```python
from build123d import *

# Parameters (mm, degrees)
SKETCH1_R                                            = 37.5
BOSS_EXTRUDE1_DEPTH                                  = 10
CSK_FOR_M6_HEX_SOCKET_COUNTERSUNK_CAP_SC_D           = 7
CSK_FOR_M6_HEX_SOCKET_COUNTERSUNK_CAP_SC_DEPTH       = 14.44
CSK_FOR_M6_HEX_SOCKET_COUNTERSUNK_CAP_SC_CSINK_D     = 13.44
CSK_FOR_M6_HEX_SOCKET_COUNTERSUNK_CAP_SC_CSINK_ANGLE = 90
CSK_FOR_M6_HEX_SOCKET_COUNTERSUNK_CAP_SC_TIP         = 2.103012167
SKETCH6_W                                            = 15
SKETCH6_H                                            = 30
BOSS_EXTRUDE2_DEPTH                                  = 7
SKETCH7_W                                            = 15
SKETCH7_H                                            = 30
BOSS_EXTRUDE3_DEPTH                                  = 7
BOSS_EXTRUDE4_START                                  = -7.5
BOSS_EXTRUDE4_DEPTH                                  = 7.5
FILLET1_R                                            = 10
SKETCH9_R                                            = 2.1
CUT_EXTRUDE1_DEPTH                                   = 6
SKETCH11_R                                           = 2.1
BOSS_EXTRUDE5_DEPTH                                  = 25
SKETCH12_W                                           = 3.472021997
SKETCH12_H                                           = 10.744400241
CUT_EXTRUDE2_DEPTH                                   = 25
BOSS_EXTRUDE7_DEPTH                                  = 10
SKETCH15_4_W                                         = 18.896565648
SKETCH15_4_H                                         = 10
BOSS_EXTRUDE8_DEPTH                                  = 27.8
F_1_4_0_25_DIAMETER_HOLE2_D                          = 6.35
F_1_4_0_25_DIAMETER_HOLE2_DEPTH                      = 15
F_1_4_0_25_DIAMETER_HOLE2_TIP                        = 1.907732465
SKETCH24_W                                           = 18.896565648
SKETCH24_H                                           = 23.705231447
BOSS_EXTRUDE9_DEPTH                                  = 11.55
FILLET2_R                                            = 10
FILLET4_R                                            = 5


with BuildPart() as part:
    # Sketch1 → Boss-Extrude1 (new body)
    with BuildSketch(Plane.XY):
        with Locations((-0.136852044, 0.136852044)):
            Circle(SKETCH1_R)
    extrude(amount=BOSS_EXTRUDE1_DEPTH)

    # CSK for M6 Hex Socket Countersunk Cap Screw1
    with Locations(Plane(origin=(0, 0, 0), x_dir=(-1, 0, 0), z_dir=(0, 0, -1))):
        with Locations((-17.388332087, 17.58954996), (-17.388332087, -17.337031875), (17.941484165, -17.337031875)):
            CounterSinkHole(CSK_FOR_M6_HEX_SOCKET_COUNTERSUNK_CAP_SC_D / 2, CSK_FOR_M6_HEX_SOCKET_COUNTERSUNK_CAP_SC_CSINK_D / 2, depth=CSK_FOR_M6_HEX_SOCKET_COUNTERSUNK_CAP_SC_DEPTH, counter_sink_angle=CSK_FOR_M6_HEX_SOCKET_COUNTERSUNK_CAP_SC_CSINK_ANGLE)
            with Locations((0, 0, -(CSK_FOR_M6_HEX_SOCKET_COUNTERSUNK_CAP_SC_DEPTH + CSK_FOR_M6_HEX_SOCKET_COUNTERSUNK_CAP_SC_TIP / 2))):  # 118° drill point
                Cone(0, CSK_FOR_M6_HEX_SOCKET_COUNTERSUNK_CAP_SC_D / 2, CSK_FOR_M6_HEX_SOCKET_COUNTERSUNK_CAP_SC_TIP, mode=Mode.SUBTRACT)



with BuildPart() as body_2:
    # Sketch6 → Boss-Extrude2 (new body)
    with BuildSketch(Plane(origin=(50, 0, 0), x_dir=(0, 0, -1), z_dir=(1, 0, 0))):
        Rectangle(SKETCH6_W, SKETCH6_H)
    extrude(amount=BOSS_EXTRUDE2_DEPTH)


with BuildPart() as body_3:
    # Sketch7 → Boss-Extrude3 (new body)
    with BuildSketch(Plane(origin=(-50, 0, 0), x_dir=(0, 0, -1), z_dir=(1, 0, 0))):
        Rectangle(SKETCH7_W, SKETCH7_H)
    extrude(amount=-BOSS_EXTRUDE3_DEPTH)


with BuildPart() as part_1:
    add(part.part)

    add(body_2.part)  # Boss-Extrude4 merges body 2

    add(body_3.part)  # Boss-Extrude4 merges body 3
    # Sketch8 → Boss-Extrude4 (add)
    with BuildSketch(Plane(origin=(0, 0, -7.5), x_dir=(-1, 0, 0), z_dir=(0, 0, -1)).offset(BOSS_EXTRUDE4_START)):
        with BuildLine():
            Line((-34.291869002, 15), (-57, 15))
            Line((-57, 15), (-57, -15))
            Line((-57, -15), (-34.172413618, -15))
            Line((-34.172413618, -15), (-23.688862383, -15))
            ThreePointArc((-23.688862383, -15), (-17.388332087, -10.617031875), (-11.087801791, -15))
            Line((-11.087801791, -15), (11.640953869, -15))
            ThreePointArc((11.640953869, -15), (17.941484165, -10.617031875), (24.242014462, -15))
            Line((24.242014462, -15), (34.446117705, -15))
            Line((34.446117705, -15), (57, -15))
            Line((57, -15), (57, 15))
            Line((57, 15), (34.565573089, 15))
            Line((34.565573089, 15), (24.142502711, 15))
            Line((24.142502711, 15), (11.74046562, 15))
            Line((11.74046562, 15), (-11.187313541, 15))
            ThreePointArc((-11.187313541, 15), (-17.388332087, 10.86954996), (-23.589350633, 15))
            Line((-23.589350633, 15), (-34.291869002, 15))
        make_face()
    extrude(amount=BOSS_EXTRUDE4_DEPTH)

    # Fillet1
    # the kernel refuses this fillet: 10 mm, written as the material it adds along each edge
    with BuildSketch(Plane(origin=(-50, -15, 0), x_dir=(0, 0, 1), z_dir=(0, 1, 0))) as fillet1_piece_1:
        with BuildLine():
            CenterArc((10, 9.682458366), FILLET1_R, 180, 75.522487814)
            Line((0, 9.682458366), (-0.2, 9.682458366))
            Line((-0.2, 9.682458366), (-0.2, 0))
            Line((-0.2, 0), (0, -0.2))
            ThreePointArc((0, -0.2), (3.75, -0.2), (7.45, -0.193649167))
            Line((7.45, -0.193649167), (7.5, 0))
        make_face()
    extrude(amount=30)
    with BuildSketch(Plane(origin=(50, -15, 0), x_dir=(0, 0, 1), z_dir=(0, 1, 0))) as fillet1_piece_2:
        with BuildLine():
            CenterArc((10, -9.682458366), FILLET1_R, 104.477512186, 75.522487814)
            Line((0, -9.682458366), (-0.2, -9.682458366))
            Line((-0.2, -9.682458366), (-0.2, 0))
            Line((-0.2, 0), (0, 0.2))
            ThreePointArc((0, 0.2), (3.75, 0.2), (7.45, 0.193649167))
            Line((7.45, 0.193649167), (7.5, 0))
        make_face()
    extrude(amount=30)

    # Sketch9 → Cut-Extrude1 (cut)
    with BuildSketch(Plane(origin=(57, 0, 0), x_dir=(0, 0, -1), z_dir=(1, 0, 0))):
        with Locations((0, -7.5)):
            Circle(SKETCH9_R)
        with Locations((0, 7.5)):
            Circle(SKETCH9_R)
    cut_extrude1 = extrude(amount=-CUT_EXTRUDE1_DEPTH, mode=Mode.SUBTRACT)

    # Mirror1: Cut-Extrude1 across plane
    add(cut_extrude1.mirror(Plane(origin=(0, 0, 0), x_dir=(0, 0, 1), z_dir=(1, 0, 0))), mode=Mode.SUBTRACT)

    # Sketch11 → Boss-Extrude5 (add)
    # profile 1 of 2: a face of its own
    with BuildSketch(Plane(origin=(0, 0, -7.5), x_dir=(-1, 0, 0), z_dir=(0, 0, -1))):
        with BuildLine():
            Line((27.636852044, 12.286852044), (27.636852044, -12.013147956))
            Line((27.636852044, -12.013147956), (31.536852044, -12.013147956))
            ThreePointArc((31.536852044, -12.013147956), (32.243958825, -11.720254738), (32.536852044, -11.013147956))
            Line((32.536852044, -11.013147956), (33.536852044, -11.013147956))
            ThreePointArc((33.536852044, -11.013147956), (35.658172387, -10.1344683), (36.536852044, -8.013147956))
            Line((36.536852044, -8.013147956), (36.536852044, -6.013147956))
            ThreePointArc((36.536852044, -6.013147956), (35.658172387, -3.891827613), (33.536852044, -3.013147956))
            Line((33.536852044, -3.013147956), (32.536852044, -3.013147956))
            Line((32.536852044, -3.013147956), (32.536852044, 3.386852044))
            Line((32.536852044, 3.386852044), (33.536852044, 3.386852044))
            ThreePointArc((33.536852044, 3.386852044), (35.658172387, 4.2655317), (36.536852044, 6.386852044))
            Line((36.536852044, 6.386852044), (36.536852044, 8.386852044))
            ThreePointArc((36.536852044, 8.386852044), (35.658172387, 10.508172387), (33.536852044, 11.386852044))
            Line((33.536852044, 11.386852044), (32.531839481, 11.386852044))
            ThreePointArc((32.531839481, 11.386852044), (32.207672437, 12.028471892), (31.536852044, 12.286852044))
            Line((31.536852044, 12.286852044), (27.636852044, 12.286852044))
        make_face()
        with Locations((32.437183431, -7.013147956)):
            Circle(SKETCH11_R, mode=Mode.SUBTRACT)
        with Locations((32.437183431, 7.386852044)):
            Circle(SKETCH11_R, mode=Mode.SUBTRACT)
    # profile 2 of 2: a face of its own
    with BuildSketch(Plane(origin=(0, 0, -7.5), x_dir=(-1, 0, 0), z_dir=(0, 0, -1))):
        with BuildLine():
            Line((0.436852044, -12.013147956), (0.436852044, -4.263147956))
            Line((0.436852044, -4.263147956), (-9.663147956, -4.263147956))
            Line((-9.663147956, -4.263147956), (-9.663147956, -8.263147956))
            ThreePointArc((-9.663147956, -8.263147956), (-9.370254738, -8.970254738), (-8.663147956, -9.263147956))
            Line((-8.663147956, -9.263147956), (-7.856041175, -9.263147956))
            Line((-7.856041175, -9.263147956), (-7.856041175, -9.656041175))
            ThreePointArc((-7.856041175, -9.656041175), (-6.977361519, -11.777361519), (-4.856041175, -12.656041175))
            Line((-4.856041175, -12.656041175), (-3.511855719, -12.656041175))
            ThreePointArc((-3.511855719, -12.656041175), (-2.52984766, -12.490765178), (-1.656041175, -12.013147956))
            Line((-1.656041175, -12.013147956), (0.436852044, -12.013147956))
        make_face()
        with Locations((-4.016957243, -8.560264433)):
            Circle(SKETCH11_R, mode=Mode.SUBTRACT)
    extrude(amount=BOSS_EXTRUDE5_DEPTH)

    # Sketch12 → Cut-Extrude2 (cut)
    with BuildSketch(Plane(origin=(0, 0, -32.5), x_dir=(-1, 0, 0), z_dir=(0, 0, -1))):
        with Locations((0.436852044, -4.263147957)):
            Rectangle(SKETCH12_W, SKETCH12_H)
    extrude(amount=-CUT_EXTRUDE2_DEPTH, mode=Mode.SUBTRACT)

    # Sketch15 → Boss-Extrude7 (add)
    with BuildSketch(Plane(origin=(0, 0, 0), x_dir=(-1, 0, 0), z_dir=(0, 0, -1))):
        with BuildLine():
            ThreePointArc((9.585134895, -36.153366351), (0.136852072, -37.363147956), (-9.311430753, -36.153366366))
            Line((-9.311430753, -36.153366366), (-9.311430753, -48.705231447))
            Line((-9.311430753, -48.705231447), (9.585134895, -48.705231447))
            Line((9.585134895, -48.705231447), (9.585134895, -36.153366351))
        make_face()
    extrude(amount=-BOSS_EXTRUDE7_DEPTH)

    # Sketch15<4> → Boss-Extrude8 (add)
    with BuildSketch(Plane(origin=(0, 0, 0), x_dir=(-1, 0, 0), z_dir=(0, 0, -1))):
        with Locations((0.136852071, -43.705231447)):
            Rectangle(SKETCH15_4_W, SKETCH15_4_H)
    extrude(amount=BOSS_EXTRUDE8_DEPTH)

    # 1/4 (0.25) Diameter Hole2
    with Locations(Plane(origin=(0, -48.705231447, 0), x_dir=(-1, 0, 0), z_dir=(0, -1, 0))):
        with Locations((0.136852046, 21.7)):
            Hole(F_1_4_0_25_DIAMETER_HOLE2_D / 2, depth=F_1_4_0_25_DIAMETER_HOLE2_DEPTH)
            with Locations((0, 0, -(F_1_4_0_25_DIAMETER_HOLE2_DEPTH + F_1_4_0_25_DIAMETER_HOLE2_TIP / 2))):  # 118° drill point
                Cone(0, F_1_4_0_25_DIAMETER_HOLE2_D / 2, F_1_4_0_25_DIAMETER_HOLE2_TIP, mode=Mode.SUBTRACT)

    # Sketch24 → Boss-Extrude9 (add)
    with BuildSketch(Plane(origin=(0, 0, 0), x_dir=(-1, 0, 0), z_dir=(0, 0, -1))):
        with Locations((0.136852071, -26.852615724)):
            Rectangle(SKETCH24_W, SKETCH24_H)
    extrude(amount=BOSS_EXTRUDE9_DEPTH)

    # Fillet2
    fillet2_edges = [part_1.edges().sort_by_distance(p)[0] for p in [
        (-9.585134895, -36.153366351, 5),
        (9.311430753, -36.153366366, 5),
    ]]
    fillet(fillet2_edges, radius=FILLET2_R)

    # Fillet4
    fillet4_edges = [part_1.edges().sort_by_distance(p)[0] for p in [
        (9.311430753, -48.705231447, -8.9),
        (-9.585134895, -48.705231447, -8.9),
        (-9.585134895, -43.705231447, -27.8),
        (9.311430753, -43.705231447, -27.8),
    ]]
    fillet(fillet4_edges, radius=FILLET4_R)


solid = part_1.part
```
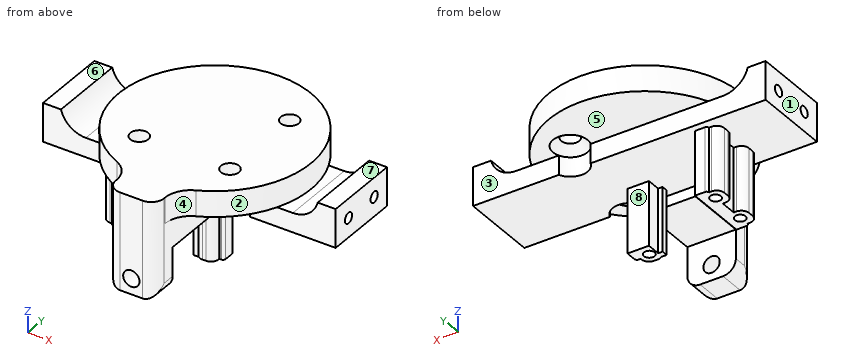
Design review of the part built by this model. Coordinates are the model's own, in mm. Face numbers are marked on the shaded views. A direction names the side the tool comes from. Coordinates: 2 decimals unless noted, no trailing zeros. Order: outer loops, then holes, each group sorted by start corner. A loop starts at its lowest first (then second) coordinate and runs counter-clockwise, first axis right, second up.
1) Take a section at B-B, the plane z = -16. State how many separate pieces and enclosed holes the cut face has, and give its area (3 significant figures).
2) Take a section at A-A, the plane y = -41. Give the boundary of the cut face in (x, z) (3 decimals).
3) Take a section at C-C, the plane y = -27.5. Give the boundary of the cut face in (x, z).
4) Wall thickness on line 1 along X through (y, z) = (6, 5.5); line 2 along X through (y, z) = (-43, -13.5); line 3 along Y through (x, z) = (-42, -3): over which ranges is each line inside the solid? List them lowest first.
5) Mouldability with a two-part tool opening along X and no side actions: class the marked faces 1, 2, 3 and 4 as +X half, -X half, draft (parallel to the pull), parting line (faces both ways), or undercut.
6) Clearance check with flat-ended pins moving along their axes: pin 1 (2 mm diameter, centred on x = -35.5, z = -15.5, fed in from -Y); pin 2 (1.5 mm diameter, centred on x = -31, z = -16.5, fed in from +Y); pin 3 (10 mm diameter, centred on x = 14, z = -20, fed in from +Y). State where each tip first meets the part, or that it passes through.
7) For the marked faces 5, 6, 7 and 8, list the 3-axis set-ups (+Z, -Z, +X, -X, +Y, -Y) from which the entire face can be reached by the end or side of a thin tool; tool diameter is ignored.
Returned:
1. separate pieces: 3
1. enclosed holes: 3
1. area: 377 mm2
2. outline: (-9.83, 0) - (-9.585, 0) - (-9.585, -22.8) arc R5 ccw to (-4.585, -27.8) - (4.311, -27.8) arc R5 ccw to (9.311, -22.8) - (9.311, 0) - (9.556, 0) - (9.556, 10) - (-9.83, 10) - close; hole circle Ø6.35 at (-0.137, -21.7)
3. outline: (-25.48, 0) - (-9.59, 0) - (-9.59, -11.55) - (9.31, -11.55) - (9.31, 0) - (25.21, 0) - (25.21, 10) - (-25.48, 10) - close
4. line 1: x = -57 to -49.25, -37.18 to 36.9, 49.25 to 57
4. line 2: x = -9.59 to 9.31
4. line 3: y = -15 to 15
5. face 1: -X half
5. face 2: undercut
5. face 3: draft
5. face 4: +X half
6. pin 1: stops at y = -10.85
6. pin 2: stops at y = 12.29
6. pin 3: stops at y = -4.26
7. face 5: -Z, +X, -X, +Y
7. face 6: +Z, -X, +Y, -Y
7. face 7: +Z, +X, +Y, -Y
7. face 8: -Z, +X, +Y
